from build123d import *

# Parameters (mm, degrees)
SKETCH1_W           = 45.999999948
SKETCH1_H           = 13.700000032
SKETCH1_R           = 1.599999975
BOSS_EXTRUDE1_DEPTH = 0.79375


with BuildPart() as part:
    # Sketch1 → Boss-Extrude1 (new body, symmetric)
    with BuildSketch(Plane(origin=(0, 0, 0), x_dir=(1, 0, 0), z_dir=(0, 1, 0))):
        Rectangle(SKETCH1_W, SKETCH1_H)
        with Locations((-19.550000016, 0)):
            Circle(SKETCH1_R, mode=Mode.SUBTRACT)
        with Locations((19.550000016, 0)):
            Circle(SKETCH1_R, mode=Mode.SUBTRACT)
    extrude(amount=BOSS_EXTRUDE1_DEPTH, both=True)


solid = part.part
For this review, take the finished solid that the model builds, in its own axes (mm). Round coordinates to 2 decimals unless told otherwise and drop trailing zeros. Loops run counter-clockwise (first coordinate to the right, second up) from the corner with the lowest first, then second, coordinate; pieces in that order, holes last. Notation, with made-up numbers: (10, 56.25) - (27, 56.25) arc R24 cw to (27, 91.25) - close; hole circle Ø3 at (-8, -30). An arc over 180 degrees is marked (long way). One line per item, written item: value. Start each with the question number.
Item 1: The part is to be moulded in two halves that separate along Z. For faces 1 (the cylindrical face through (17.95, -0.01, -0.07)), 2 (the flat face through (0, 0, 6.85)), 3 (the flat face through (0, 0, -6.85)), 4 (the flat face through (0, -0.794, 0)), say which applies: +Z half, -Z half, draft (parallel to the pull), parting line (faces both ways), or undercut.
Item 2: For L1, parallel to X at y = 0.1, z = 0; L2, parallel to Z at x = -19.55, y = -0.3; L3, parallel to X at y = -0.55, z = -1, list the stretches that pass through material, from the lowest coordinate up.
Item 3: Take a section at B-B (x = 19.55). Give the boundary of the cut face in (y, z), plus the area to 3 significant figures.
Item 4: Take a section at A-A (z = 0). Give the boundary of the cut face in (x, y).
Item 5: Take a section at C-C (y = 0.1). Give the boundary of the cut face in (x, z).
Item 6: Clearance check with a flat-ended pin moving along its axis: pin 1 Ø2.5 at (x, z) = (-19.55, 0) entering from -Y. State where the tip first meets the part, or that it passes through.
Answer below:
1. face 1: undercut
1. face 2: +Z half
1. face 3: -Z half
1. face 4: draft
2. L1: x = -23 to -21.15, -17.95 to 17.95, 21.15 to 23
2. L2: z = -6.85 to -1.6, 1.6 to 6.85
2. L3: x = -23 to -20.8, -18.3 to 18.3, 20.8 to 23
3. outline: (-0.79, -6.85) - (0.79, -6.85) - (0.79, -1.6) - (-0.79, -1.6) - close; (-0.79, 1.6) - (0.79, 1.6) - (0.79, 6.85) - (-0.79, 6.85) - close
3. area: 16.7 mm2
4. outline: (-23, -0.79) - (-21.15, -0.79) - (-21.15, 0.79) - (-23, 0.79) - close; (-17.95, -0.79) - (17.95, -0.79) - (17.95, 0.79) - (-17.95, 0.79) - close; (21.15, -0.79) - (23, -0.79) - (23, 0.79) - (21.15, 0.79) - close
5. outline: (-23, -6.85) - (23, -6.85) - (23, 6.85) - (-23, 6.85) - close; hole circle Ø3.2 at (-19.55, 0); hole circle Ø3.2 at (19.55, 0)
6. pin 1: passes through
